Could you check a few things on this model? Use its own coordinates, in mm. A direction names the side the tool comes from. Round coordinates to 2 decimals unless told otherwise and drop trailing zeros. Loops run counter-clockwise (first coordinate to the right, second up) from the corner with the lowest first, then second, coordinate; pieces in that order, holes last. Notation, with made-up numbers: M -0.5,12 L 50.5,12 A26 cw 50.5,50 Z; hole C -18,61 d9. An arc over 180 degrees is marked long. Answer in a Markdown table with one row per item.
```python
from build123d import *

# Parameters (mm, degrees)
F0_R        = 3.75
F0_R_2      = 1.75
F0_R_3      = 0.9
F1_DEPTH    = 6
F0_R_4      = 6
F1_FACE_R   = 3.75
F1_FACE_R_2 = 0.9
F2_DEPTH    = 6
F3_START    = 8
F3_DEPTH    = 6
F4_SIZE     = 0.5
F5_SIZE     = 0.2
F6_SIZE     = 0.5


with BuildPart() as f1:
    # F0 (on Top) → F1 (new body)
    with BuildSketch(Plane.XY):
        Circle(F0_R)
        Circle(F0_R_2, mode=Mode.SUBTRACT)
        Circle(F0_R_2)
        Circle(F0_R_3, mode=Mode.SUBTRACT)
    extrude(amount=F1_DEPTH)

    # F0 (on Top) + F1_face (on face) → F2 (join)
    with BuildSketch(Plane.XY):
        Circle(F0_R_4)
        Circle(F0_R, mode=Mode.SUBTRACT)
    with BuildSketch(Plane.XY.offset(6)):
        Circle(F1_FACE_R)
        Circle(F1_FACE_R_2, mode=Mode.SUBTRACT)
    extrude(amount=F2_DEPTH)

    # F0 (on Top) → F3 (cut)
    with BuildSketch(Plane.XY.offset(F3_START)):
        Circle(F0_R_2)
        Circle(F0_R_3, mode=Mode.SUBTRACT)
    extrude(amount=F3_DEPTH, mode=Mode.SUBTRACT)

    # F4
    f4_edges = [f1.edges().sort_by_distance(p)[0] for p in [
        (-0.9, 0, 0),
    ]]
    chamfer(f4_edges, length=F4_SIZE)

    # F5
    f5_edges = [f1.edges().sort_by_distance(p)[0] for p in [
        (-6, 0, 6),
    ]]
    chamfer(f5_edges, length=F5_SIZE)

    # F6
    f6_edges = [f1.edges().sort_by_distance(p)[0] for p in [
        (-3.75, 0, 12),
        (-1.75, 0, 12),
    ]]
    chamfer(f6_edges, length=F6_SIZE)


solid = f1.part
```
1) I need wall thicknesses on line 1 (Y direction, x = 0, z = 2.5); line 2 (Z direction, x = -3, y = 3); line 3 (X direction, y = -0.5, z = 8.25). Which ranges of each line are inside material? Lowest first, please.
Computed:
| item | result |
|---|---|
| line 1 | y = -6 to -0.9, 0.9 to 6 |
| line 2 | z = 0 to 6 |
| line 3 | x = -3.72 to -1.68, 1.68 to 3.72 |
2) Will these pins go through, and if not, where does the flat tip stop? P1, Ø3, axis at y = 5, z = 6, coming from the +X side; P2, Ø3, axis at x = 0.5, y = -0.5, coming from the +Z side; P3, Ø2, axis at y = -3, z = 10.5, coming from the -X side.
Computed:
| item | result |
|---|---|
| P1 | stops at x = 4.86 |
| P2 | stops at z = 11.96 |
| P3 | stops at x = -3.17 |
3) I want a section at A-A, the plane x = 0. Please give me the cut outline in (y, z).
Computed:
| item | result |
|---|---|
| outline | M -6,0 L -1.4,0 L -0.9,0.5 L -0.9,8 L -1.75,8 L -1.75,11.5 L -2.25,12 L -3.25,12 L -3.75,11.5 L -3.75,6 L -5.8,6 L -6,5.8 Z; M 0.9,0.5 L 1.4,0 L 6,0 L 6,5.8 L 5.8,6 L 3.75,6 L 3.75,11.5 L 3.25,12 L 2.25,12 L 1.75,11.5 L 1.75,8 L 0.9,8 Z |
4) I want a section at C-C, the plane z = 10.5. Please give me the cut outline in (x, y).
Computed:
| item | result |
|---|---|
| outline | C 0,0 d7.5; hole C 0,0 d3.5 |
5) I want a section at D-D, the plane z = 4. Please give me the cut outline in (x, y), plus the area to 3 significant figures.
Computed:
| item | result |
|---|---|
| outline | C 0,0 d12; hole C 0,0 d1.8 |
| area | 111 mm² |
6) Which directions (+Z, -Z, +X, -X, +Y, -Y) give clear straight access to the entire face, cutting with the end or side of a thin tool? Please do faces 5 (the face through (-6, 0, 3)), 6 (the face through (1, -1, 8)).
Computed:
| item | result |
|---|---|
| face 5 | +Z, -Z |
| face 6 | +Z |
7) If we mould it in two halves opening along Y, with no side actions, what happens to faces 1 (the face through (1.2, -1.2, 0)), 2 (the face through (0.86, 0.27, 4.2)), 3 (the face through (1.617, -0.67, 9.726)), 4 (the face through (-3.746, 0.165, 8.712))? For each: released by +Y, released by -Y, zero draft, split by the parting line, or undercut.
Computed:
| item | result |
|---|---|
| face 1 | zero draft |
| face 2 | undercut |
| face 3 | undercut |
| face 4 | split by the parting line |
